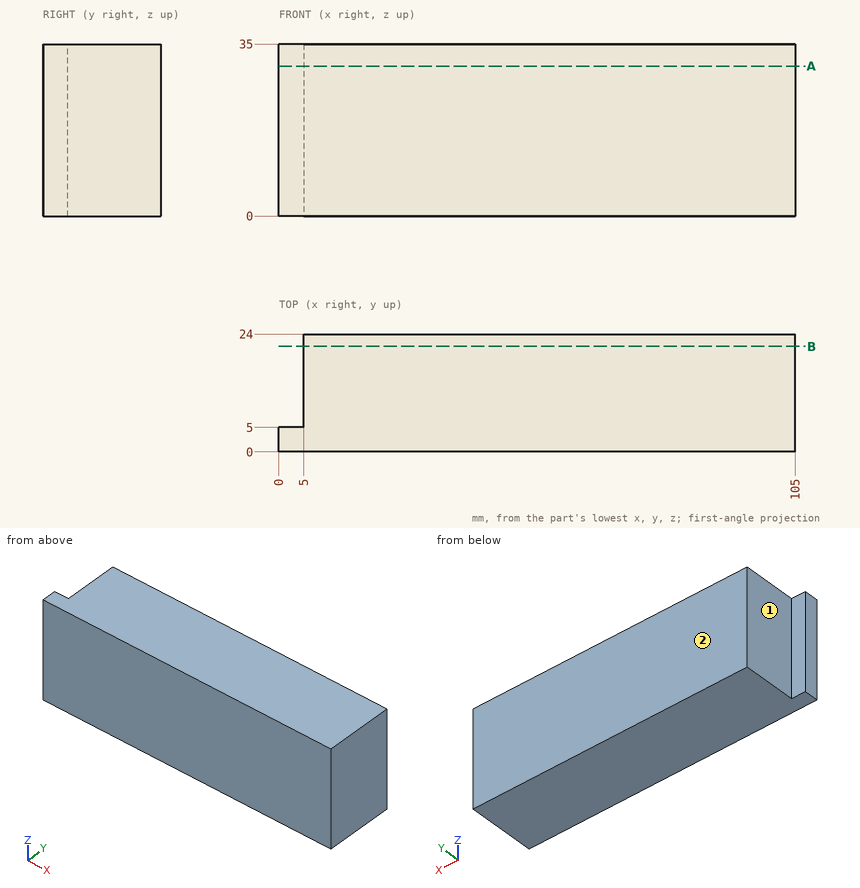
Source: three-view drawing plus pictorial views. Frame: mm from the lowest corner of the part. A direction names the side the tool comes from. Give positions to 0.01 mm unless a question says otherwise; leave off trailing zeros. Order: outer loops, then holes, each group sorted by start corner. A loop starts at its lowest first (then second) coordinate and runs counter-clockwise, first axis right, second up. Notation, with made-up numbers: M -17,44 L 12,44 A11 cw 12,48 Z; hole C 48,74.5 d11. An arc over 180 degrees is marked long. One line per question, with ' | ' between items. Start each with the question number.
1. First-contact query: pin 1 Ø9.5 at (y, z) = (18, 25.5) entering from -X; pin 2 Ø1.5 at (x, z) = (1.5, 11) entering from +Y. Flat tips, straight axial feed; report the tip coordinate or a pass-through.
2. Access query for the marked faces 1 and 2. Directions: +Z, -Z, +X, -X, +Y, -Y. A direction counts if a zero-diameter tool reaches every point of the face in a straight line with its end or side. Return the directions, or none.
3. Material intervals for probe 1 along X at (y, z) = (6, 33), sorted ascending. Write a range as [from, to].
4. Section query A-A (z = 30.5). Return the cut outline in (x, y).
5. Section query B-B (y = 21.5). Return the cut outline in (x, z).
Here are the results:
1) pin 1: x = 5 | pin 2: y = 5
2) face 1: +Z, -Z, -X, +Y | face 2: +Z, -Z, +X, -X, +Y
3) probe 1: [5, 105]
4) outline: M 0,0 L 105,0 L 105,24 L 5,24 L 5,5 L 0,5 Z
5) outline: M 5,0 L 105,0 L 105,35 L 5,35 Z
